from build123d import *

# Parameters (mm, degrees)
BOSS_EXTRUDE1_DEPTH           = 3.7
CHAMFER1_SIZE                 = 1.5
SKETCH2_R                     = 3
BOSS_EXTRUDE2_DEPTH           = 3
BOSS_EXTRUDE2_DRAFT           = 10
BOSS_EXTRUDE2_PROFILE_2_DEPTH = 3
BOSS_EXTRUDE2_PROFILE_2_DRAFT = 10
BOSS_EXTRUDE2_PROFILE_3_DEPTH = 3
BOSS_EXTRUDE2_PROFILE_3_DRAFT = 10


with BuildPart() as part:
    # Sketch1 → Boss-Extrude1 (new body)
    with BuildSketch(Plane.XY):
        Polygon((100, 7.893729842), (-100, 7.893729842), (-93.951405808, -7.416270158), (93.951405808, -7.416270158), align=None)
    extrude(amount=BOSS_EXTRUDE1_DEPTH)

    # Chamfer1
    chamfer1_edges = [part.edges().sort_by_distance(p)[0] for p in [
        (0, 7.893729842, 3.7),
        (-96.975702904, 0.238729842, 3.7),
        (0, -7.416270158, 3.7),
        (96.975702904, 0.238729842, 3.7),
    ]]
    chamfer(chamfer1_edges, length=CHAMFER1_SIZE)


with BuildPart() as boss_extrude2_tool:
    # Sketch2 → Boss-Extrude2 (with draft: the straight prism first)
    with BuildSketch(Plane(origin=(0, 0, 0), x_dir=(-1, 0, 0), z_dir=(0, 0, -1))):
        with Locations((-69.740425787, 1.006073404)):
            Circle(SKETCH2_R)
    extrude(amount=BOSS_EXTRUDE2_DEPTH)
    # Boss-Extrude2: the draft: its side faces are tilted about the plane it starts from
    boss_extrude2_sides = [boss_extrude2_tool.faces().sort_by_distance(p)[0] for p in [
        (72.740425787, 1.006073404, -1.5),
    ]]
    draft(boss_extrude2_sides, Plane(origin=(0, 0, 0), x_dir=(-1, 0, 0), z_dir=(0, 0, -1)), BOSS_EXTRUDE2_DRAFT)


with BuildPart() as part_1:
    add(part.part)

    # Boss-Extrude2: add boss_extrude2_tool
    add(boss_extrude2_tool.part)


with BuildPart() as boss_extrude2_profile_2_tool:
    # Sketch2 → Boss-Extrude2 profile 2 (with draft: the straight prism first)
    with BuildSketch(Plane(origin=(0, 0, 0), x_dir=(-1, 0, 0), z_dir=(0, 0, -1))):
        with Locations((0.259574213, 1.006073404)):
            Circle(SKETCH2_R)
    extrude(amount=BOSS_EXTRUDE2_PROFILE_2_DEPTH)
    # Boss-Extrude2 profile 2: the draft: its side faces are tilted about the plane it starts from
    boss_extrude2_profile_2_sides = [boss_extrude2_profile_2_tool.faces().sort_by_distance(p)[0] for p in [
        (2.740425787, 1.006073404, -1.5),
    ]]
    draft(boss_extrude2_profile_2_sides, Plane(origin=(0, 0, 0), x_dir=(-1, 0, 0), z_dir=(0, 0, -1)), BOSS_EXTRUDE2_PROFILE_2_DRAFT)


with BuildPart() as part_2:
    add(part_1.part)

    # Boss-Extrude2 profile 2: add boss_extrude2_profile_2_tool
    add(boss_extrude2_profile_2_tool.part)


with BuildPart() as boss_extrude2_profile_3_tool:
    # Sketch2 → Boss-Extrude2 profile 3 (with draft: the straight prism first)
    with BuildSketch(Plane(origin=(0, 0, 0), x_dir=(-1, 0, 0), z_dir=(0, 0, -1))):
        with Locations((70.259574213, 1.006073404)):
            Circle(SKETCH2_R)
    extrude(amount=BOSS_EXTRUDE2_PROFILE_3_DEPTH)
    # Boss-Extrude2 profile 3: the draft: its side faces are tilted about the plane it starts from
    boss_extrude2_profile_3_sides = [boss_extrude2_profile_3_tool.faces().sort_by_distance(p)[0] for p in [
        (-67.259574213, 1.006073404, -1.5),
    ]]
    draft(boss_extrude2_profile_3_sides, Plane(origin=(0, 0, 0), x_dir=(-1, 0, 0), z_dir=(0, 0, -1)), BOSS_EXTRUDE2_PROFILE_3_DRAFT)


with BuildPart() as part_3:
    add(part_2.part)

    # Boss-Extrude2 profile 3: add boss_extrude2_profile_3_tool
    add(boss_extrude2_profile_3_tool.part)


solid = part_3.part
Check sheet for the modelled part. Datum: model origin and axes. Units: mm. Round coordinates to 2 decimals unless told otherwise and drop trailing zeros. Loops run counter-clockwise (first coordinate to the right, second up) from the corner with the lowest first, then second, coordinate; pieces in that order, holes last.
1. Scan lines: probe 1 along X at (y, z) = (1, -1); probe 2 along Z at (x, y) = (36, -1.5); probe 3 along X at (y, z) = (-1, 2.25). Record each from-to range of solid material in increasing order.
2. Sectioned sample at A-A on x = -26.5. Record the boundary of the cut face in (y, z), and give its area (3 significant figures).
3. Sectioned sample at B-B on z = -1.75. Record the boundary of the cut face in (x, y).
4. Mould release check, pull along X, two halves, no side actions. Record for faces 1 (the flat face through (-96.311, 0.625, 2.96)), 2 (the conical face through (67.184, 1.811, -1.812)), 3 (the flat face through (96.226, 0.411, 2.96)): released by +X, released by -X, zero draft, split by the parting line, or undercut.
5. Gauge pin test, flat end, axial feed: pin 1 Ø2 at (x, y) = (71, -5) entering from -Z. Record the tip position at first contact, or that the pin passes through.
Recorded:
1. probe 1: x = -73.08 to -67.44, -3.08 to 2.56, 66.92 to 72.56
1. probe 2: z = 0 to 3.7
1. probe 3: x = -96.43 to 96.43
2. outline: (-7.42, 0) - (7.89, 0) - (7.89, 2.2) - (6.39, 3.7) - (-5.92, 3.7) - (-7.42, 2.2) - close
2. area: 54.4 mm2
3. outline: circle Ø5.38 at (-70.26, 1.01); circle Ø5.38 at (-0.26, 1.01); circle Ø5.38 at (69.74, 1.01)
4. face 1: released by -X
4. face 2: undercut
4. face 3: released by +X
5. pin 1: stops at z = 0
